Autodesk Inventor part; units mm, degrees
ref_plane "YZ Plane" through (0, 0, 0) normal (1, 0, 0) x (0, 1, 0)
ref_plane "XZ Plane" through (0, 0, 0) normal (0, 1, 0) x (-1, 0, 0)
ref_plane "XY Plane" through (0, 0, 0) normal (0, 0, 1) x (1, 0, 0)
sketch "Body Outline" plane through (0, 0, 0) normal (0, 1, 0) x (-1, 0, 0)
  line L0 (54.5, -6) -> (-54.5, -6)
  line L1 (-54.5, -6) -> (-54.5, 6)
  line L2 (-54.5, 6) -> (54.5, 6)
  line L3 (54.5, 6) -> (54.5, -6)
  point P0 (0, 0)
  dimension "d0" = 109
  dimension "d1" = 54.5
  dimension "d2" = 12
  dimension "d3" = 6
extrude "Body" add sketch "Body Outline" along normal blind 6
sketch "Clamp Cutout Outline" plane through (54.5, 0, 6) normal (1, 0, 0) x (0, 0, -1)
  line L0 (2, 7.3) -> (10, 7.3)
  line L1 (10, 7.3) -> (10, 5.3)
  line L2 (10, 5.3) -> (2, 5.3)
  line L3 (2, 5.3) -> (2, 7.3)
  line L4 (0, 6) -> (12, 6)
  line L5 (0, 0) -> (0, 6)
  line L6 (12, 0) -> (12, 6)
  point P0 (6, 0)
  dimension "d6" = 0.7
  dimension "d7" = 2
  dimension "d8" = 2
  dimension "d9" = 2
extrude "Clamp Cutout" cut sketch "Clamp Cutout Outline" along normal through all both and the other way through all
sketch "Fastening Hole Positions" plane through (0, 0, 0) normal (0, -1, 0) x (1, 0, 0)
  point P0 (0, 0)
  point P1 (20, 0)
  point P2 (0, 0)
  point P3 (-20, 0)
  point P4 (45, 0)
  point P5 (-45, 0)
  dimension "d12" = 20
  dimension "d13" = 20
  dimension "d14" = 0
  dimension "d15" = 0
  dimension "d16" = 0
  dimension "d17" = 0
  dimension "d26" = 25
  dimension "d27" = 25
  dimension "d28" = 0
  dimension "d29" = 0
hole "Fastening Holes" at (20, 0, 0) at (0, 0, 0) at (-20, 0, 0) at (-45, 0, 0) at (45, 0, 0) direction (0, 1, 0) diameter 5.2 end through all countersink diameter 11 countersink angle 90
equation "\"d8\" = d7"
properties part number "LR Large Clamp" material "Aluminum 6061"
Can you work these out from the model? Positions are in its coordinate system, mm. A direction names the side the tool comes from. Round coordinates to 2 decimals unless told otherwise and drop trailing zeros. Loops run counter-clockwise (first coordinate to the right, second up) from the corner with the lowest first, then second, coordinate; pieces in that order, holes last. Notation, with made-up numbers: (-3, 61.5) -> (29, 61.5) arc R15 cw to (29, 80.5) -> close; hole circle Ø5 at (17.5, -16). An arc over 180 degrees is marked (long way). One line per item, written item: value. Start each with the question number.
1. For faces 5 (the flat face through (1, 5.3, -3)), 6 (the conical face through (-19.16, 2.72, -2.65)), which set-ups out of +Z, -Z, +X, -X, +Y, -Y let a thin tool reach every point of the face, with its end or its side?
2. If we section it at A-A, the plane z = 0: Give the number of separate pieces and of enclosed holes in the cut face, then the cut area to 3 significant figures.
3. If we section it at C-C, the plane y = 4.3: Write out the boundary of the cut face in (x, z).
4. For pin 1 (4 mm diameter, centred on x = 0, z = 0, fed in from +Y); pin 2 (7 mm diameter, centred on x = -45, z = 0, fed in from +Y); pin 3 (1.5 mm diameter, centred on x = -13.5, z = -3, fed in from -Y); pin 4 (6 mm diameter, centred on x = -20, z = 0, fed in from -Y), each with a flat end and sliding along its axis, tell me the tip position at first contact or that it passes through.
5. If we mould it in two halves opening along X, with no side actions, what happens to faces 1 (the flat face through (13, 0, 0)), 2 (the flat face through (54.5, 3, 0)), 3 (the flat face through (-54.5, 3, 0)), 4 (the cylindrical face through (-42.46, 4.12, 0.56))? For each: pulls with the +X half, pulls with the -X half, needs draft (parallel to the pull), parting line crosses it, or undercut.
6. If we section it at B-B, the plane x = 20: Write out the boundary of the cut face in (y, z).
7. If I drill on probe 1 along X at (y, z) = (4.3, 0); probe 2 along Z at (x, y) = (-2, 5.55); probe 3 along X at (y, z) = (0.65, -2), over which ranges is the centre line in solid material (lowest first)?
8. If we section it at D-D, the plane x = 8: Write out the boundary of the cut face in (y, z).
Calculated:
1. face 5: +X, -X, +Y
1. face 6: -Y
2. separate pieces: 6
2. enclosed holes: 0
2. area: 398 mm²
3. outline: (-54.5, -6) -> (54.5, -6) -> (54.5, 6) -> (-54.5, 6) -> close; hole circle Ø5.2 at (-45, 0); hole circle Ø5.2 at (-20, 0); hole circle Ø5.2 at (0, 0); hole circle Ø5.2 at (20, 0); hole circle Ø5.2 at (45, 0)
4. pin 1: passes through
4. pin 2: stops at y = 5.3
4. pin 3: stops at y = 0
4. pin 4: stops at y = 2.5
5. face 1: needs draft
5. face 2: pulls with the +X half
5. face 3: pulls with the -X half
5. face 4: undercut
6. outline: (0, -6) -> (6, -6) -> (6, -4) -> (5.3, -4) -> (5.3, -2.6) -> (2.9, -2.6) -> (0, -5.5) -> close; (0, 5.5) -> (2.9, 2.6) -> (5.3, 2.6) -> (5.3, 4) -> (6, 4) -> (6, 6) -> (0, 6) -> close
7. probe 1: x = -54.5 to -47.6, -42.4 to -22.6, -17.4 to -2.6, 2.6 to 17.4, 22.6 to 42.4, 47.6 to 54.5
7. probe 2: z = -6 to -4, 4 to 6
7. probe 3: x = -54.5 to -49.42, -40.58 to -24.42, -15.58 to -4.42, 4.42 to 15.58, 24.42 to 40.58, 49.42 to 54.5
8. outline: (0, -6) -> (6, -6) -> (6, -4) -> (5.3, -4) -> (5.3, 4) -> (6, 4) -> (6, 6) -> (0, 6) -> close
